Read the model definition and answer for the solid it produces. Units are mm, in the model's axes. Coordinates: 2 decimals unless noted, no trailing zeros. Write each loop counter-clockwise with the first axis right and the second up, starting at its lowest first coordinate (ties: lowest second). Pieces come first, ordered by that corner, then holes.
1) Each of these flat-tipped pins is pushed along its axis until it touches: pin 1 Ø5 at (y, z) = (4, 18.5) entering from -X; pin 2 Ø4.5 at (x, z) = (-16.69, 51.36) entering from +Y; pin 3 Ø3 at (y, z) = (6.5, -51) entering from -X. Where does it stop, or does it pass through?
2) The part is cut by section D-D (x = 0). Determine the outline of the cut face in (y, z).
3) The part is cut by section A-A (z = 0). Determine the outline of the cut face in (x, y), then the cut area to 3 significant figures.
4) The part is cut by section B-B (x = 54). Determine the outline of the cut face in (y, z).
5) Find the intervals of material crossed by line 1 (Z direction, x = 15, y = 1.25); line 2 (Y direction, x = 55, z = -8); line 3 (Z direction, x = 54, y = 5.25), in increasing order.
Autodesk Inventor part; units mm, degrees
ref_plane "YZ Plane" through (0, 0, 0) normal (1, 0, 0) x (0, 1, 0)
ref_plane "XZ Plane" through (0, 0, 0) normal (0, 1, 0) x (-1, 0, 0)
ref_plane "XY Plane" through (0, 0, 0) normal (0, 0, 1) x (1, 0, 0)
sketch "Sketch1" plane through (0, 0, 0) normal (0, 1, 0) x (-1, 0, 0)
  circle A0 centre (0, 0) radius 65
  dimension "d0" = 130
extrude "Extrusion1" add sketch "Sketch1" along normal blind 7
sketch "Sketch5" plane through (0, 7, 0) normal (0, 1, 0) x (1, 0, 0)
  circle A0 centre (0, 0) radius 6
  dimension "d27" = 12
extrude "Extrusion5" add sketch "Sketch5" along normal blind 2
sketch "Sketch7" plane through (0, 0, 0) normal (0, -1, 0) x (1, 0, 0)
  circle A0 centre (0, 0) radius 65
  line L0 (0, 0) -> (54, 0)
  circle A1 centre (54, 0) radius 2
  dimension "d37" = 4
  dimension "d38" = 54
extrude "Extrusion7" cut sketch "Sketch7" against normal blind 10 contours A1
pattern_circular "Circular Pattern1" count 10 over 360 about axis through (0, 0, 0) along (0, -1, 0) of "Extrusion7"
properties part number "bay container 10 bottom"
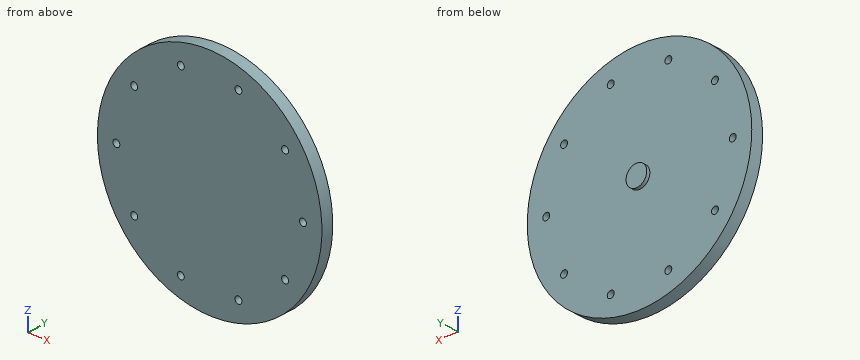
Reported:
1. pin 1: stops at x = -63
1. pin 2: stops at y = 7
1. pin 3: stops at x = -42.13
2. outline: (0, -65) - (7, -65) - (7, -6) - (9, -6) - (9, 6) - (7, 6) - (7, 65) - (0, 65) - close
3. outline: (-65, 0) - (-56, 0) - (-56, 7) - (-65, 7) - close; (-52, 0) - (52, 0) - (52, 7) - (6, 7) - (6, 9) - (-6, 9) - (-6, 7) - (-52, 7) - close; (56, 0) - (65, 0) - (65, 7) - (56, 7) - close
3. area: 878 mm2
4. outline: (0, -36.18) - (7, -36.18) - (7, -2) - (0, -2) - close; (0, 2) - (7, 2) - (7, 36.18) - (0, 36.18) - close
5. line 1: z = -63.25 to -52.43, -50.28 to 50.28, 52.43 to 63.25
5. line 2: y = 0 to 7
5. line 3: z = -36.18 to -2, 2 to 36.18
